```python
from build123d import *

# Parameters (mm, degrees)
SKETCH_1_W      = 50
SKETCH_1_H      = 6
SKETCH_1_R      = 1.75
SKETCH_1_R_2    = 1.162790698
EXTRUDE_1_DEPTH = 4
FILLET_1_R      = 3


with BuildPart() as part:
    # 草圖1 → 填料-伸長1 (new body)
    with BuildSketch(Plane(origin=(0, 0, 0), x_dir=(1, 0, 0), z_dir=(0, 1, 0))):
        Rectangle(SKETCH_1_W, SKETCH_1_H)
        with Locations(Location((-19, 0, 0), (0, 0, 270))):
            Circle(SKETCH_1_R, mode=Mode.SUBTRACT)
        with Locations(Location((19, 0, 0), (0, 0, 270))):
            Circle(SKETCH_1_R, mode=Mode.SUBTRACT)
        with Locations(Location((-13.062015504, 0, 0), (0, 0, 270))):
            Circle(SKETCH_1_R_2, mode=Mode.SUBTRACT)
        with Locations(Location((-10.062015504, 0, 0), (0, 0, 270))):
            Circle(SKETCH_1_R_2, mode=Mode.SUBTRACT)
        with Locations(Location((-7.062015504, 0, 0), (0, 0, 270))):
            Circle(SKETCH_1_R_2, mode=Mode.SUBTRACT)
        with Locations(Location((-4.062015504, 0, 0), (0, 0, 270))):
            Circle(SKETCH_1_R_2, mode=Mode.SUBTRACT)
        with Locations(Location((-1.062015504, 0, 0), (0, 0, 270))):
            Circle(SKETCH_1_R_2, mode=Mode.SUBTRACT)
        with Locations(Location((1.937984496, 0, 0), (0, 0, 270))):
            Circle(SKETCH_1_R_2, mode=Mode.SUBTRACT)
        with Locations(Location((4.937984496, 0, 0), (0, 0, 270))):
            Circle(SKETCH_1_R_2, mode=Mode.SUBTRACT)
        with Locations(Location((7.937984496, 0, 0), (0, 0, 270))):
            Circle(SKETCH_1_R_2, mode=Mode.SUBTRACT)
        with Locations(Location((10.937984496, 0, 0), (0, 0, 270))):
            Circle(SKETCH_1_R_2, mode=Mode.SUBTRACT)
        with Locations(Location((13.937984496, 0, 0), (0, 0, 270))):
            Circle(SKETCH_1_R_2, mode=Mode.SUBTRACT)
    extrude(amount=EXTRUDE_1_DEPTH)

    # 圓角1
    fillet_1_edges = [part.edges().sort_by_distance(p)[0] for p in [
        (25, 2, 3),
        (25, 2, -3),
        (-25, 2, -3),
        (-25, 2, 3),
    ]]
    fillet(fillet_1_edges, radius=FILLET_1_R - 0.0001)  # a hair under: the kernel refuses the full size


solid = part.part
```
Could you check a few things on this model? Use its own coordinates, in mm. Round coordinates to 2 decimals unless told otherwise and drop trailing zeros. Order: outer loops, then holes, each group sorted by start corner. A loop starts at its lowest first (then second) coordinate and runs counter-clockwise, first axis right, second up. Notation, with made-up numbers: M -34,14.5 L -13,14.5 A21 ccw -13,50.5 Z; hole C -10.75,24 d10. An arc over 180 degrees is marked long. One line per question, with ' | ' between items. Start each with the question number.
(1) Thinking about a two-plate mould opening in Z: for faces 1 (the face through (0, 4, 1)), 2 (the face through (24.1, 2.03, 2.14)), 3 (the face through (-3.71, 1.97, 1.11)), which applies, +Z half, -Z half, draft (parallel to the pull), parting line (faces both ways), or undercut?
(2) Suppose I cut it at B-B on y = 2.4. Count the separate pieces of the cut face and the enclosed holes in it, then the cut area to 3 significant figures.
(3) Suppose I cut it at A-A on x = 19. List the corners of the cut face in (y, z) for me.
(4) Suppose I cut it at C-C on z = 2.5. List the corners of the cut face in (x, y) for me, then the cut area to 3 significant figures.
(5) Please list where these lines run through material, in increasing order: line 1 along X through (y, z) = (3.5, -1.5); line 2 along X through (y, z) = (3.55, 1.25); line 3 along Z through (x, y) = (19.5, 0.3).
(6) For P1, Ø1, axis at y = 1, z = -1.5, coming from the -X side, with a flat end and sliding along its axis, tell me the tip position at first contact or that it passes through.
Geometry results:
1) face 1: draft | face 2: +Z half | face 3: undercut
2) separate pieces: 1 | enclosed holes: 12 | area: 231 mm²
3) outline: M 0,-3 L 4,-3 L 4,-1.75 L 0,-1.75 Z; M 0,1.75 L 4,1.75 L 4,3 L 0,3 Z
4) outline: M -23.66,0 L 23.66,0 L 23.66,4 L -23.66,4 Z | area: 189 mm²
5) line 1: -24.6 to -19.9, -18.1 to 18.1, 19.9 to 24.6 | line 2: -24.73 to -20.22, -17.78 to 17.78, 20.22 to 24.73 | line 3: -3 to -1.68, 1.68 to 3
6) P1: x = -24.83
